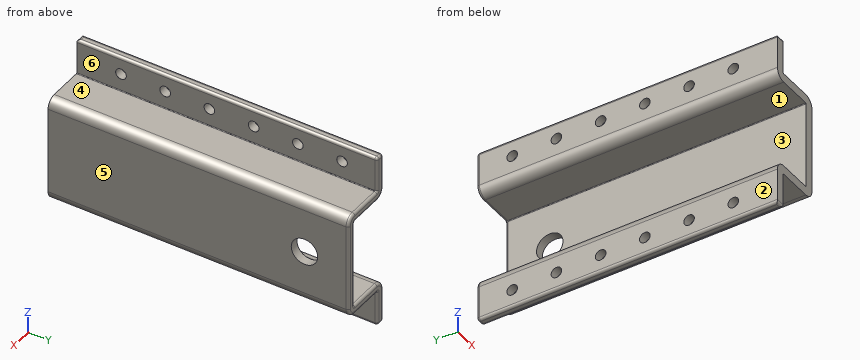
```python
from build123d import *

# Parameters (mm, degrees)
SKETCH1_W                       = 120
SKETCH1_H                       = 340
BASE_FLANGE1_DEPTH              = 10
EDGE_FLANGE1_STRIP_W            = 41.4732
EDGE_FLANGE1_STRIP_H            = 10
EDGE_FLANGE1_STRIP_CUT_DEPTH    = 340
EDGE_FLANGE1_STRIP_2_W          = 41.4732
EDGE_FLANGE1_STRIP_2_H          = 10
EDGE_FLANGE1_STRIP_CUT_2_DEPTH  = 340
EDGE_FLANGE1_DEPTH              = 340
EDGE_FLANGE1_BEND_DEPTH         = 340
EDGE_FLANGE2_STRIP_W            = 41.4732
EDGE_FLANGE2_STRIP_H            = 10
EDGE_FLANGE2_STRIP_CUT_DEPTH    = 340
EDGE_FLANGE2_STRIP_2_W          = 41.4732
EDGE_FLANGE2_STRIP_2_H          = 10
EDGE_FLANGE2_STRIP_CUT_2_DEPTH  = 340
EDGE_FLANGE2_DEPTH              = 340
EDGE_FLANGE2_BEND_DEPTH         = 340
SKETCH18_R                      = 15
CUT_EXTRUDE1_DEPTH              = 207.155281281
M10_CLEARANCE_HOLE1_D           = 12
M10_CLEARANCE_HOLE1_CSINK_D     = 12.05
M10_CLEARANCE_HOLE1_CSINK_ANGLE = 90
FILLET1_R                       = 3


# Sheet-metal steps are written as plain solids
with BuildPart() as part:
    # Sketch1 → Base-Flange1 (new body)
    with BuildSketch(Plane(origin=(0, 0, 0), x_dir=(0, 0, -1), z_dir=(1, 0, 0))):
        Rectangle(SKETCH1_W, SKETCH1_H)
    extrude(amount=BASE_FLANGE1_DEPTH)

    # Edge-Flange1 strip (across the edge) → Edge-Flange1 strip cut (cut)
    with BuildSketch(Plane(origin=(0, -170, 60), x_dir=(0, 0, -1), z_dir=(0, 1, 0))):
        with Locations((-10, -5)):
            Rectangle(EDGE_FLANGE1_STRIP_W, EDGE_FLANGE1_STRIP_H)
    extrude(amount=EDGE_FLANGE1_STRIP_CUT_DEPTH, mode=Mode.SUBTRACT)

    # Edge-Flange1 strip 2 (across the edge) → Edge-Flange1 strip cut 2 (cut)
    with BuildSketch(Plane(origin=(0, 170, -60), x_dir=(0, 0, 1), z_dir=(0, -1, 0))):
        with Locations((-10, -5)):
            Rectangle(EDGE_FLANGE1_STRIP_2_W, EDGE_FLANGE1_STRIP_2_H)
    extrude(amount=EDGE_FLANGE1_STRIP_CUT_2_DEPTH, mode=Mode.SUBTRACT)

    # Edge-Flange1 section (across the edge) → Edge-Flange1 (add)
    with BuildSketch(Plane(origin=(0, -170, 60), x_dir=(0, 0, -1), z_dir=(0, 1, 0))):
        with BuildLine():
            Line((0, 0.7366), (0, 50))
            Line((0, 50), (10, 50))
            Line((10, 50), (10, 0.7366))
            ThreePointArc((10, 0.7366), (10.215745145, 0.215745145), (10.7366, 0))
            Line((10.7366, 0), (10.7366, -10))
            ThreePointArc((10.7366, -10), (3.144677333, -6.855322667), (0, 0.7366))
        make_face()
    extrude(amount=EDGE_FLANGE1_DEPTH)

    # Edge-Flange1 section 2 (across the edge) → Edge-Flange1 bend (add)
    with BuildSketch(Plane(origin=(0, 170, -60), x_dir=(0, 0, 1), z_dir=(0, -1, 0))):
        with BuildLine():
            Line((0, 0.7366), (0, 50))
            Line((0, 50), (10, 50))
            Line((10, 50), (10, 0.7366))
            ThreePointArc((10, 0.7366), (10.215745145, 0.215745145), (10.7366, 0))
            Line((10.7366, 0), (10.7366, -10))
            ThreePointArc((10.7366, -10), (3.144677333, -6.855322667), (0, 0.7366))
        make_face()
    extrude(amount=EDGE_FLANGE1_BEND_DEPTH)

    # Edge-Flange2 strip (across the edge) → Edge-Flange2 strip cut (cut)
    with BuildSketch(Plane(origin=(-50, 170, 60), x_dir=(1, 0, 0), z_dir=(0, -1, 0))):
        with Locations((-10, -5)):
            Rectangle(EDGE_FLANGE2_STRIP_W, EDGE_FLANGE2_STRIP_H)
    extrude(amount=EDGE_FLANGE2_STRIP_CUT_DEPTH, mode=Mode.SUBTRACT)

    # Edge-Flange2 strip 2 (across the edge) → Edge-Flange2 strip cut 2 (cut)
    with BuildSketch(Plane(origin=(-50, -170, -60), x_dir=(1, 0, 0), z_dir=(0, 1, 0))):
        with Locations((-10, -5)):
            Rectangle(EDGE_FLANGE2_STRIP_2_W, EDGE_FLANGE2_STRIP_2_H)
    extrude(amount=EDGE_FLANGE2_STRIP_CUT_2_DEPTH, mode=Mode.SUBTRACT)

    # Edge-Flange2 section (across the edge) → Edge-Flange2 (add)
    with BuildSketch(Plane(origin=(-50, 170, 60), x_dir=(1, 0, 0), z_dir=(0, -1, 0))):
        with BuildLine():
            Line((0, 0.7366), (0, 40))
            Line((0, 40), (10, 40))
            Line((10, 40), (10, 0.7366))
            ThreePointArc((10, 0.7366), (10.215745145, 0.215745145), (10.7366, 0))
            Line((10.7366, 0), (10.7366, -10))
            ThreePointArc((10.7366, -10), (3.144677333, -6.855322667), (0, 0.7366))
        make_face()
    extrude(amount=EDGE_FLANGE2_DEPTH)

    # Edge-Flange2 section 2 (across the edge) → Edge-Flange2 bend (add)
    with BuildSketch(Plane(origin=(-50, -170, -60), x_dir=(1, 0, 0), z_dir=(0, 1, 0))):
        with BuildLine():
            Line((0, 0.7366), (0, 40))
            Line((0, 40), (10, 40))
            Line((10, 40), (10, 0.7366))
            ThreePointArc((10, 0.7366), (10.215745145, 0.215745145), (10.7366, 0))
            Line((10.7366, 0), (10.7366, -10))
            ThreePointArc((10.7366, -10), (3.144677333, -6.855322667), (0, 0.7366))
        make_face()
    extrude(amount=EDGE_FLANGE2_BEND_DEPTH)

    # Sketch18 → Cut-Extrude1 (cut, through all)
    with BuildSketch(Plane(origin=(10, 0, 0), x_dir=(0, 0, -1), z_dir=(1, 0, 0))):
        with Locations((0, 120)):
            Circle(SKETCH18_R)
    extrude(amount=-CUT_EXTRUDE1_DEPTH, mode=Mode.SUBTRACT)

    # M10 Clearance Hole1 (through all)
    with Locations(Plane(origin=(-40, 0, 0), x_dir=(0, 0, -1), z_dir=(1, 0, 0))):
        with Locations((80, -120), (80, -70), (80, -20), (80, 30), (80, 80), (80, 130)):
            m10_clearance_hole1 = CounterSinkHole(M10_CLEARANCE_HOLE1_D / 2, M10_CLEARANCE_HOLE1_CSINK_D / 2, counter_sink_angle=M10_CLEARANCE_HOLE1_CSINK_ANGLE)

    # Mirror1: M10 Clearance Hole1 across plane
    add(m10_clearance_hole1.mirror(Plane.XY), mode=Mode.SUBTRACT)

    # Fillet1
    fillet1_edges = [part.edges().sort_by_distance(p)[0] for p in [
        (-46.855322667, 170, 53.144677333),
        (-39.784254855, 170, 60.215745145),
        (-45, 170, 100),
        (-40, 170, 80.3683),
        (-50, 0, 100),
        (-50, 170, 80.3683),
        (-40, 0, 100),
        (-45, -170, 100),
        (-46.855322667, 170, -53.144677333),
        (-39.784254855, 170, -60.215745145),
        (-45, -170, -100),
        (-40, 170, -80.3683),
        (-50, 170, -80.3683),
        (-50, 0, -100),
        (-40, 0, -100),
        (-45, 170, -100),
        (0, 170, 0),
        (10, 170, 0),
        (6.855322667, 170, 56.855322667),
        (-0.215745145, 170, 49.784254855),
        (-20, 170, 50),
        (-20, 170, 60),
        (6.855322667, 170, -56.855322667),
        (-0.215745145, 170, -49.784254855),
        (-20, 170, -50),
        (-20, 170, -60),
    ]]
    fillet(fillet1_edges, radius=FILLET1_R)


solid = part.part
```
The model under review builds one solid part; all positions refer to its coordinate system, in mm. Face numbers are marked on the shaded views. A direction names the side the tool comes from. Give positions to 0.01 mm unless a question says otherwise; leave off trailing zeros. Write each loop counter-clockwise with the first axis right and the second up, starting at its lowest first coordinate (ties: lowest second). Pieces come first, ordered by that corner, then holes.
(1) Consider section D-D, the plane y = -57. Give the boundary of the cut face in (x, z), and give its area (3 significant figures).
(2) To check wall thickness, follow L1, parallel to Z at x = -33, y = 5; L2, parallel to Z at x = -45.75, y = 130; L3, parallel to Z at x = -44, y = -70. State the ranges of each line that lie inside material, in increasing order.
(3) Consider section A-A, the plane z = 0. Give the boundary of the cut face in (x, y), and give its area (3 significant figures).
(4) For P1, Ø11.5, axis at x = -29, y = 5, coming from the +Z side; P2, Ø15.5, axis at y = 130, z = -80, coming from the +X side; P3, Ø12, axis at y = 24, z = -41, coming from the -X side, all flat-tipped, find the tip position at first contact; note any pin that passes through.
(5) The part is to be moulded in two halves that separate along Z. For the marked faces 1, 2, 3 and 4, say which applies: released by +Z, released by -Z, zero draft, split by the parting line, or undercut.
(6) Tool access review of the marked faces 5 and 6: name each direction out of +Z, -Z, +X, -X, +Y, -Y from which nothing blocks a thin tool from reaching the whole face with its end or side.
(7) Consider section C-C, the plane y = 120. Give the boundary of the cut face in (x, z).
(8) Consider section B-B, the plane x = -27. Give the boundary of the cut face in (y, z).
Returned:
1. outline: (-50, -97) arc R3 ccw to (-47, -100) - (-43, -100) arc R3 ccw to (-40, -97) - (-40, -60.74) arc R0.74 cw to (-39.26, -60) - (-0.74, -60) arc R10.74 ccw to (10, -49.26) - (10, 49.26) arc R10.74 ccw to (-0.74, 60) - (-39.26, 60) arc R0.74 cw to (-40, 60.74) - (-40, 97) arc R3 ccw to (-43, 100) - (-47, 100) arc R3 ccw to (-50, 97) - (-50, 60.74) arc R10.74 ccw to (-39.26, 50) - (-0.74, 50) arc R0.74 cw to (0, 49.26) - (0, -49.26) arc R0.74 cw to (-0.74, -50) - (-39.26, -50) arc R10.74 ccw to (-50, -60.74) - close
1. area: 2,890 mm2
2. L1: z = -60 to -50, 50 to 60
2. L2: z = -100 to -86, -74 to -52.18, 52.18 to 74, 86 to 100
2. L3: z = -100 to -86, -74 to -51.1, 51.1 to 74, 86 to 100
3. outline: (0, -170) - (10, -170) - (10, 105) - (0, 105) - close; (0, 135) - (10, 135) - (10, 167) arc R3 ccw to (7, 170) - (3, 170) arc R3 ccw to (0, 167) - close
3. area: 3,100 mm2
4. P1: stops at z = 60
4. P2: stops at x = -40
4. P3: stops at x = 0
5. face 1: undercut
5. face 2: zero draft
5. face 3: undercut
5. face 4: released by +Z
6. face 5: +Z, -Z, +X, +Y, -Y
6. face 6: +Z, +X, +Y, -Y
7. outline: (-50, -97) arc R3 ccw to (-47, -100) - (-43, -100) arc R3 ccw to (-40, -97) - (-40, -60.74) arc R0.74 cw to (-39.26, -60) - (-0.74, -60) arc R10.74 ccw to (10, -49.26) - (10, -15) - (0, -15) - (0, -49.26) arc R0.74 cw to (-0.74, -50) - (-39.26, -50) arc R10.74 ccw to (-50, -60.74) - close; (-50, 60.74) arc R10.74 ccw to (-39.26, 50) - (-0.74, 50) arc R0.74 cw to (0, 49.26) - (0, 15) - (10, 15) - (10, 49.26) arc R10.74 ccw to (-0.74, 60) - (-39.26, 60) arc R0.74 cw to (-40, 60.74) - (-40, 97) arc R3 ccw to (-43, 100) - (-47, 100) arc R3 ccw to (-50, 97) - close
8. outline: (-170, -60) - (167, -60) arc R3 ccw to (170, -57) - (170, -53) arc R3 ccw to (167, -50) - (-170, -50) - close; (-170, 50) - (167, 50) arc R3 ccw to (170, 53) - (170, 57) arc R3 ccw to (167, 60) - (-170, 60) - close
